For this review, take the finished solid that the model builds, in its own axes (mm). A direction names the side the tool comes from. Round coordinates to 2 decimals unless told otherwise and drop trailing zeros. Loops run counter-clockwise (first coordinate to the right, second up) from the corner with the lowest first, then second, coordinate; pieces in that order, holes last.
1) Take a section at D-D (y = -12.5). State the section outline as (x, z) points.
2) Mouldability with a two-part tool opening along X and no side actions: class faces 1 (the cylindrical face through (-64.09, 14.4, 3.45)), 2 (the flat face through (-62, 9.5, 3)), 3 (the flat face through (-24, 4.5, -3)) as pulls with the +X half, pulls with the -X half, needs draft (parallel to the pull), parting line crosses it, or undercut.
3) Wall thickness on L1, parallel to Y at x = -78, z = 2; L2, parallel to X at y = 1, z = 5; L3, parallel to Y at x = -26, z = 6: over which ranges is each line inside the solid? List them lowest first.
4) Take a section at C-C (z = 2.75). State the section outline as (x, y) points.
5) Take a section at A-A (x = -78). State the section outline as (y, z) points.
6) Take a section at B-B (y = 0). State the section outline as (x, z) points.
7) Insertion check: pin 1 (1.5 mm diameter, centred on y = 0.5, z = -0.5, fed in from +X); pin 2 (7.5 mm diameter, centred on x = -28, z = 4, fed in from -Y); pin 3 (5.5 mm diameter, centred on x = -36, z = -2, fed in from +Y); pin 4 (5.5 mm diameter, centred on x = -18.5, z = -4, fed in from -Y). Each pin has a flat end and moves straight along its axis. Give the tip position at first contact, or say it passes through.
8) Tool access review of faces 4 (the flat face through (-51, -10, 3)), 5 (the flat face through (-24, -4.5, -3)), 6 (the flat face through (-62, -9.5, 3)): name each direction out of +Z, -Z, +X, -X, +Y, -Y from which nothing blocks a thin tool from reaching the whole face with its end or side.
```python
from build123d import *

# Parameters (mm, degrees)
PAD_DEPTH         = 7
PAD001_DEPTH      = 7
POCKET_DEPTH      = 7.001
POCKET_DEPTH_BACK = 7.001


with BuildPart() as part:
    # Sketch → Pad (new body)
    with BuildSketch(Plane.XY):
        with BuildLine():
            Line((-51, 9), (0, 9))
            ThreePointArc((0, -9), (9, 0), (0, 9))
            Line((-51, -9), (0, -9))
            Line((-51, -11.5), (-51, -9))
            ThreePointArc((-53.5, -14), (-51.732233, -13.267767), (-51, -11.5))
            Line((-61.667517, -14), (-53.5, -14))
            ThreePointArc((-61.667517, -14), (-64.061085, -14.392199), (-66.204318, -15.527778))
            ThreePointArc((-66.204318, 15.527778), (-97.5, 0), (-66.204318, -15.527778))
            ThreePointArc((-66.204318, 15.527778), (-64.061085, 14.392199), (-61.667517, 14))
            Line((-61.667517, 14), (-53.5, 14))
            ThreePointArc((-51, 11.5), (-51.732233, 13.267767), (-53.5, 14))
            Line((-51, 11.5), (-51, 9))
        make_face()
        with BuildLine():
            Line((-65.719426, 9.5), (-58.219426, 9.5))
            ThreePointArc((-57.219426, 8.5), (-57.512319, 9.207107), (-58.219426, 9.5))
            Line((-57.219426, 8.5), (-57.219426, -8.5))
            ThreePointArc((-58.219426, -9.5), (-57.512319, -9.207107), (-57.219426, -8.5))
            Line((-58.219426, -9.5), (-65.719426, -9.5))
            ThreePointArc((-65.719426, -9.5), (-67.162406, -9.769342), (-68.411059, -10.541096))
            ThreePointArc((-68.411059, 10.541096), (-92.25, 0), (-68.411059, -10.541096))
            ThreePointArc((-68.411059, 10.541096), (-67.162406, 9.769342), (-65.719426, 9.5))
        make_face(mode=Mode.SUBTRACT)
    extrude(amount=PAD_DEPTH)

    # Sketch001 → Pad001 (join)
    with BuildSketch(Plane.XY):
        with BuildLine():
            Line((-54.205771, 4.5), (-54.205771, -4.5))
            Line((-54.205771, -4.5), (7.794229, -4.5))
            ThreePointArc((7.794229, -4.5), (9, 0), (7.794229, 4.5))
            Line((-54.205771, 4.5), (7.794229, 4.5))
        make_face()
    extrude(amount=-PAD001_DEPTH)

    # Sketch002 → Pocket (cut, two sides)
    with BuildSketch(Plane.XY) as pocket_sk:
        with BuildLine():
            Line((-2, 1.5), (-2, -1.5))
            ThreePointArc((-2, -1.5), (2.5, 0), (-2, 1.5))
        make_face()
    extrude(amount=-POCKET_DEPTH, mode=Mode.SUBTRACT)
    extrude(pocket_sk.sketch, amount=POCKET_DEPTH_BACK, mode=Mode.SUBTRACT)


solid = part.part
```
Response:
1. outline: (-92.97, 0) - (-84.84, 0) - (-84.84, 7) - (-92.97, 7) - close; (-71.16, 0) - (-51.21, 0) - (-51.21, 7) - (-71.16, 7) - close
2. face 1: pulls with the +X half
2. face 2: undercut
2. face 3: needs draft
3. L1: y = -19.5 to -14.25, 14.25 to 19.5
3. L2: x = -97.47 to -92.21, -57.22 to -2, 2.29 to 8.94
3. L3: y = -9 to 9
4. outline: (-66.2, -15.53) arc R7.5 cw to (-61.67, -14) - (-53.5, -14) arc R2.5 ccw to (-51, -11.5) - (-51, -9) - (0, -9) arc R9 ccw to (0, 9) - (-51, 9) - (-51, 11.5) arc R2.5 ccw to (-53.5, 14) - (-61.67, 14) arc R7.5 cw to (-66.2, 15.53) arc R19.5 ccw (long way) to start; hole (-68.41, -10.54) arc R4 cw to (-65.72, -9.5) - (-58.22, -9.5) arc R1 ccw to (-57.22, -8.5) - (-57.22, 8.5) arc R1 ccw to (-58.22, 9.5) - (-65.72, 9.5) arc R4 cw to (-68.41, 10.54) arc R14.25 ccw (long way) to start; hole (-2, -1.5) arc R2.5 ccw (long way) to (-2, 1.5) - close
5. outline: (-19.5, 0) - (-14.25, 0) - (-14.25, 7) - (-19.5, 7) - close; (14.25, 0) - (19.5, 0) - (19.5, 7) - (14.25, 7) - close
6. outline: (-97.5, 0) - (-92.25, 0) - (-92.25, 7) - (-97.5, 7) - close; (-57.22, 0) - (-54.21, 0) - (-54.21, -7) - (-2, -7) - (-2, 7) - (-57.22, 7) - close; (2.5, -7) - (9, -7) - (9, 7) - (2.5, 7) - close
7. pin 1: stops at x = 9
7. pin 2: stops at y = -9
7. pin 3: stops at y = 9
7. pin 4: stops at y = -4.5
8. face 4: +Z, -Z, +X, -Y
8. face 5: -Z, +X, -X, -Y
8. face 6: +Z, -Z
